Here's how the part is built. I have some questions about the finished solid (model axes, mm). Round coordinates to 2 decimals unless told otherwise and drop trailing zeros. Write each loop counter-clockwise with the first axis right and the second up, starting at its lowest first coordinate (ties: lowest second). Pieces come first, ordered by that corner, then holes. Notation, with made-up numbers: (76.5, 15) -> (93.5, 15) arc R6 ccw to (93.5, 24) -> close; hole circle Ø6 at (77.5, -18.75). An arc over 180 degrees is marked (long way). Put each result on its own line as item: value. Start each with the question number.
1. I need wall thicknesses on probe 1 along X at (y, z) = (130, 12.75); probe 2 along Y at (x, z) = (63, 8); probe 3 along Y at (x, z) = (52, 19). Which ranges of each line are inside material? Lowest first, please. Write a range as from..to.
2. Suppose I cut it at A-A (z = 23.25). Please give me the cut outline in (x, y).
3. For pin 1 (1 mm diameter, centred on x = 50, z = 10, fed in from +Y); pin 2 (10 mm diameter, centred on x = 64, z = 19, fed in from +Y); pin 3 (6 mm diameter, centred on y = 180.5, z = 8.5, fed in from +X), each with a flat end and sliding along its axis, tell me the tip position at first contact or that it passes through.
4. Suppose I cut it at B-B (y = 107.5). Please give me the cut outline in (x, z).
```python
from build123d import *

# Parameters (mm, degrees)
F2_DEPTH = 25.4
F3_R     = 25.39999


# Not quite as in the source:
# - a fillet or chamfer is up to 0.001 mm smaller than in the source, because OpenCascade refuses the exact size


with BuildPart() as f2:
    # F1 (on face) → F2 (new body)
    with BuildSketch(Plane.XY):
        with BuildLine():
            Line((0, 121.2334576344), (0, 80.8223050896))
            Line((0, 80.8223050896), (116.1005682623, 196.9228733519))
            ThreePointArc((116.1005682623, 196.9228733519), (102.889252487, 204.1366251379), (89.2318353651, 210.4652929995))
            Line((89.2318353651, 210.4652929995), (0, 121.2334576344))
        make_face()
    extrude(amount=F2_DEPTH)

    # F3 (radius 25.4 in the source; OpenCascade refuses exactly that, so slightly less here)
    f3_edges = [f2.edges().sort_by_distance(p)[0] for p in [
        (102.889252, 204.136625, 25.4),
    ]]
    fillet(f3_edges, radius=F3_R)


solid = f2.part
```
Verdict:
1. probe 1: x = 8.77..49.18
1. probe 2: y = 143.82..184.23
1. probe 3: y = 132.82..173.23
2. outline: (0, 80.82) -> (104.99, 185.82) arc R213.43 ccw to (77.59, 198.82) -> (0, 121.23) -> close
3. pin 1: stops at y = 171.73
3. pin 2: stops at y = 190.23
3. pin 3: stops at x = 102.68
4. outline: (0, 0) -> (26.68, 0) -> (26.68, 25.4) -> (0, 25.4) -> close
